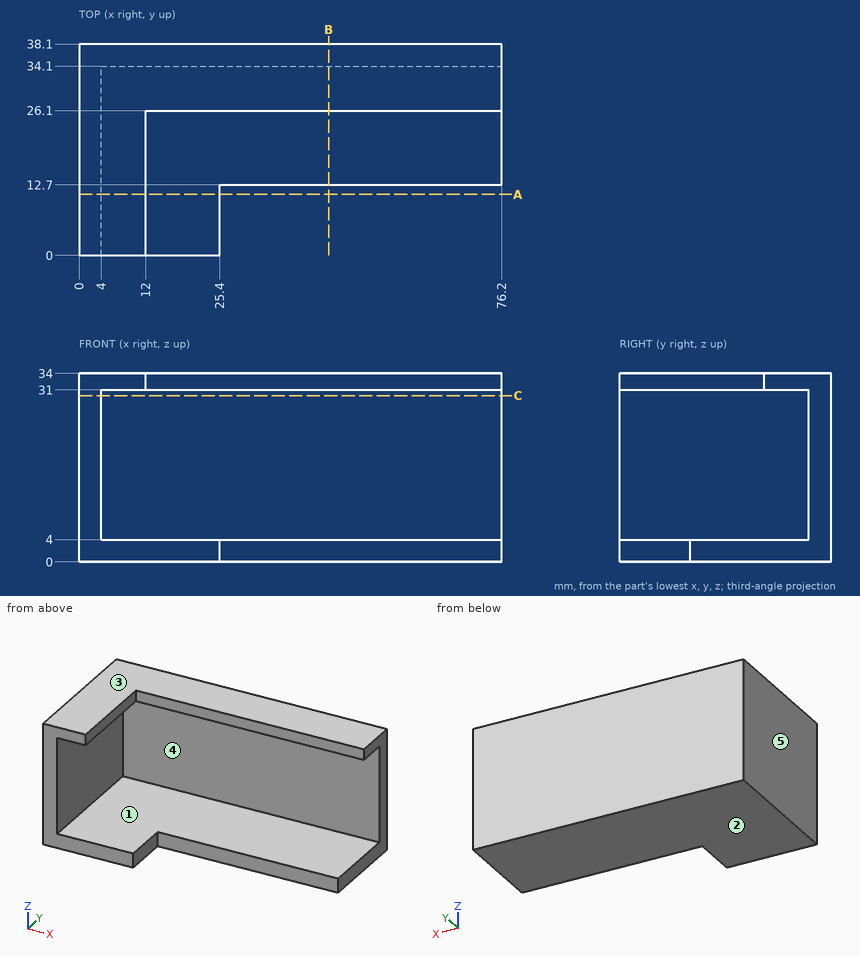
Could you check a few things on this drawing? It's one solid part, dimensions in mm from its lowest x, y, z. A direction names the side the tool comes from. Round coordinates to 2 decimals unless told otherwise and drop trailing zeros. Order: outer loops, then holes, each group sorted by start corner. A loop starts at its lowest first (then second) coordinate and runs counter-clockwise, first axis right, second up. Notation, with made-up numbers: M -39,-39 L -27,-39 A26 ccw -27,-3 Z; hole C 70,-12 d9. An arc over 180 degrees is marked long. One line per question, with ' | ' between items.
1) On a 3-axis mill with a long thin cutter (end or side, diameter ignored), from which of +Z, -Z, +X, -X, +Y, -Y can I reach the whole of each face in a straight line? I mean the marked faces 1 and 2. Say none if no direction works.
Checked values:
face 1: +X, -Y | face 2: -Z, +X, -X, +Y, -Y
2) I'm going to push flat-ended pins straight in: pin 1 Ø0.9 at (x, z) = (45.5, 32.5) entering from -Y; pin 2 Ø12 at (x, y) = (27, 20) entering from +Z; pin 3 Ø5 at (y, z) = (26, 26.5) entering from +X. Where does each tip first touch, or does it pass through?
Checked values:
pin 1: stops at y = 26.1 | pin 2: stops at z = 4 | pin 3: stops at x = 4
3) Imagine slicing it at A-A, the plane y = 11. Write out the boundary of the cut face in (x, z).
Checked values:
outline: M 0,0 L 25.4,0 L 25.4,4 L 4,4 L 4,31 L 12,31 L 12,34 L 0,34 Z
4) Imagine slicing it at C-C, the plane z = 30. Write out the boundary of the cut face in (x, y).
Checked values:
outline: M 0,0 L 4,0 L 4,34.1 L 76.2,34.1 L 76.2,38.1 L 0,38.1 Z
5) I need wall thicknesses on line 1 (Z direction, x = 8, y = 27.5); line 2 (X direction, y = 2, z = 5). Which ranges of each line are inside material? Lowest first, please.
Checked values:
line 1: z = 0 to 4, 31 to 34 | line 2: x = 0 to 4
6) We'd pull the mould along Z, two halves only. Please class the marked faces 3, 4 and 5: released by +Z, released by -Z, zero draft, split by the parting line, or undercut.
Checked values:
face 3: released by +Z | face 4: undercut | face 5: zero draft
7) Imagine slicing it at B-B, the plane x = 45. Write out the boundary of the cut face in (y, z), plus the area to 3 significant figures.
Checked values:
outline: M 12.7,0 L 38.1,0 L 38.1,34 L 26.1,34 L 26.1,31 L 34.1,31 L 34.1,4 L 12.7,4 Z | area: 246 mm²
